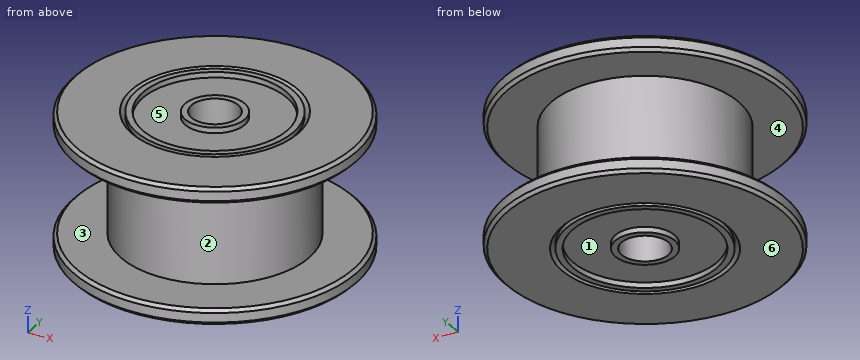
from build123d import *


with BuildPart() as part:
    # Эскиз1 → Повернуть1 (revolve)
    with BuildSketch(Plane(origin=(0, 0, 0), x_dir=(1, 0, 0), z_dir=(0, 1, 0))):
        Polygon((4.6, 4.35), (4.6, 4), (1.9, 4), (1.9, 4.35), (1.5, 4.35), (1.5, -4.35), (1.9, -4.35), (1.9, -4), (4.6, -4), (4.6, -4.35), (5, -4.35), (5, -4.05), (5.3, -4.35), (8.8, -4.35), (9, -4.15), (9, -3.55), (8.8, -3.35), (6, -3.35), (6, 3.35), (8.8, 3.35), (9, 3.55), (9, 4.15), (8.8, 4.35), (5.3, 4.35), (5, 4.05), (5, 4.35), align=None)
    revolve(axis=Axis((0, 0, -4.35), (0, 0, 1)))


solid = part.part
Check sheet for the modelled part. Datum: model origin and axes. Units: mm. Face numbers are marked on the shaded views. A direction names the side the tool comes from. Round coordinates to 2 decimals unless told otherwise and drop trailing zeros. Order: outer loops, then holes, each group sorted by start corner. A loop starts at its lowest first (then second) coordinate and runs counter-clockwise, first axis right, second up.
(1) Scan lines: probe 1 along Z at (x, y) = (-6, -5.5); probe 2 along Z at (x, y) = (-1.5, -1.25); probe 3 along Y at (x, z) = (1, -2.5). Record each from-to range of solid material in increasing order.
(2) Go/stop test with flat-tipped pins: P1, Ø8.5, axis at x = 0, y = 0, coming from the -Z side; P2, Ø2, axis at x = -1, z = 0, coming from the +Y side; P3, Ø4, axis at x = -5.5, z = 2, coming from the +Y side; P4, Ø3, axis at y = -1.5, z = -1.5, coming from the -X side. Record where each tip stops, or that it passes through.
(3) Draft check along Y on the marked faces 1, 2 and 3. Enter one of: pulls with the +Y half, pulls with the -Y half, needs draft (parallel to the pull), parting line crosses it, or undercut.
(4) Cross-section at A-A, the plane z = -1.5. Enter the section's corners in (x, y), and give its area (3 significant figures).
(5) Access from +Z, -Z, +X, -X, +Y, -Y to the whole of each face (thin tool, end or side, straight path). Record for the marked faces 4, 5 and 6.
Check sheet entries:
1. probe 1: z = -4.35 to -3.35, 3.35 to 4.35
1. probe 2: z = -4 to 4
1. probe 3: y = -5.92 to -1.12, 1.12 to 5.92
2. P1: stops at z = -4.35
2. P2: stops at y = 6
2. P3: stops at y = 7.94
2. P4: stops at x = -6
3. face 1: undercut
3. face 2: parting line crosses it
3. face 3: needs draft
4. outline: circle Ø12 at (0, 0); hole circle Ø3 at (0, 0)
4. area: 106 mm2
5. face 4: none
5. face 5: +Z
5. face 6: -Z, +X, -X, +Y, -Y
